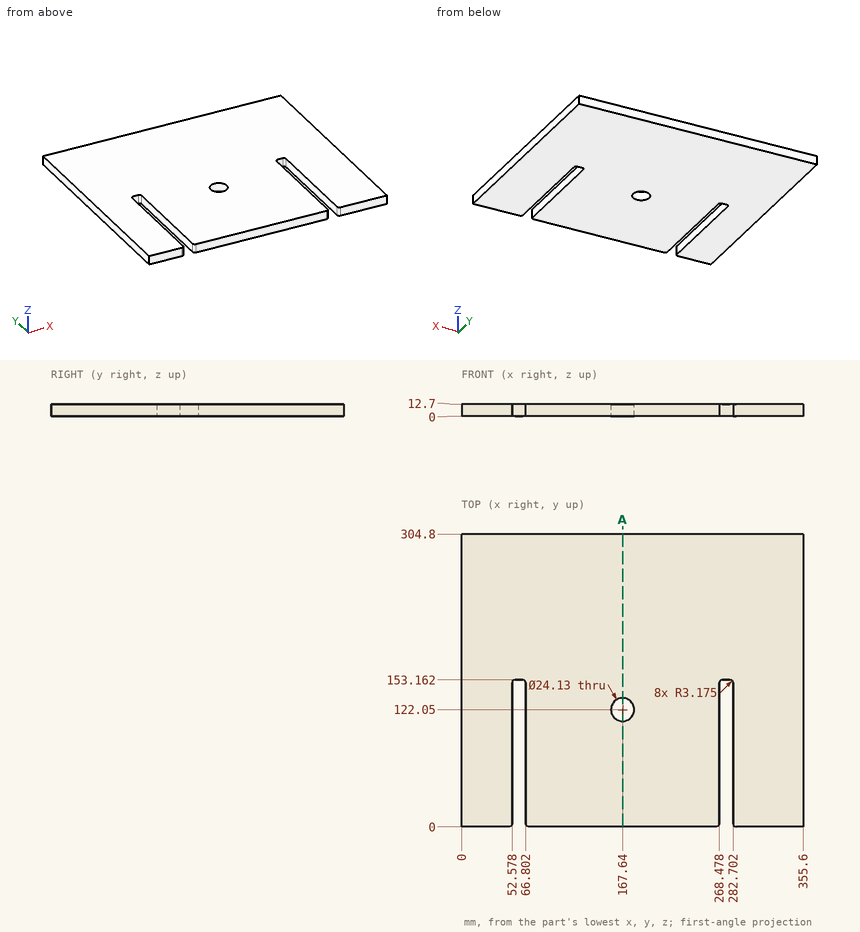
Job drawing, mm, ordinate dimensions from the low corner. One solid piece. Coordinates: 2 decimals unless noted, no trailing zeros. Write each loop counter-clockwise with the first axis right and the second up, starting at its lowest first coordinate (ties: lowest second). Pieces come first, ordered by that corner, then holes. Notation, with made-up numbers: (19, 83) - (51, 83) arc R30 ccw to (51, 114) - close; hole circle Ø1 at (5.25, 22). An arc over 180 degrees is marked (long way). Use a Markdown table: item, result. Add a question column.
Item 1: Flat gauge pins, fed straight in: pin 1 (1 mm diameter, centred on x = 267, z = 5.5, fed in from -Y) (1 decimal); pin 2 (2.5 mm diameter, centred on x = 274, z = 4.5, fed in from -Y). Where does each tip first touch, or does it go through?
Item 2: Band-saw the part on A-A, the plane x = 167.64. Give the cut face in (y, z) (1 decimal).
Item 3: Drill centre lines: L1, parallel to X at y = 106, z = 9.5; L2, parallel to Y at x = 167.64, z = 7.5 (1 decimal); L3, parallel to X at y = 130, z = 0.5 (1 decimal). Where is each one in solid material? Low to high. Write a range as from..to.
Numbers:
| question | item | result |
|---|---|---|
| 1 | pin 1 | y = 0.2 |
| 1 | pin 2 | y = 153.16 |
| 2 | outline | (0, 0) - (110, 0) - (110, 12.7) - (0, 12.7) - close; (134.1, 0) - (304.8, 0) - (304.8, 12.7) - (134.1, 12.7) - close |
| 3 | L1 | 0..52.58, 66.8..268.48, 282.7..355.6 |
| 3 | L2 | 0..110, 134.1..304.8 |
| 3 | L3 | 0..52.6, 66.8..158.6, 176.7..268.5, 282.7..355.6 |
